The figure shows three views and two pictorial views of one solid part (mm, origin at its lowest corner). Answer the questions. Round coordinates to 2 decimals unless told otherwise and drop trailing zeros. Order: outer loops, then holes, each group sorted by start corner. A loop starts at its lowest first (then second) coordinate and runs counter-clockwise, first axis right, second up. Notation, with made-up numbers: (54.25, 88.25) - (81.25, 88.25) arc R22 ccw to (81.25, 96.25) - close; hole circle Ø1 at (17, 39). An arc over 180 degrees is marked (long way). Use CSV: the item, a comma, the result in double quotes. Start each with the question number.
Item 1: Find section B-B, the plane y = 44. Give the vertices of the cut face in (x, z).
Item 2: Find section A-A, the plane z = 0.65. Give the vertices of the cut face in (x, y), plus the area to 3 significant figures.
Item 3: Find section C-C, the plane x = 65. Give the vertices of the cut face in (y, z).
Item 4: Straight lines are drawn through the part: line 1 along X through (y, z) = (45, 2.55); line 2 along X through (y, z) = (63.5, 0.6); line 3 along Y through (x, z) = (15, 3.05). For each, find the intervals that lie inside material, in ascending order. Write a range as [from, to].
Item 5: Find section D-D, the plane y = 63.5. Give the vertices of the cut face in (x, z), plus the area to 3 significant figures.
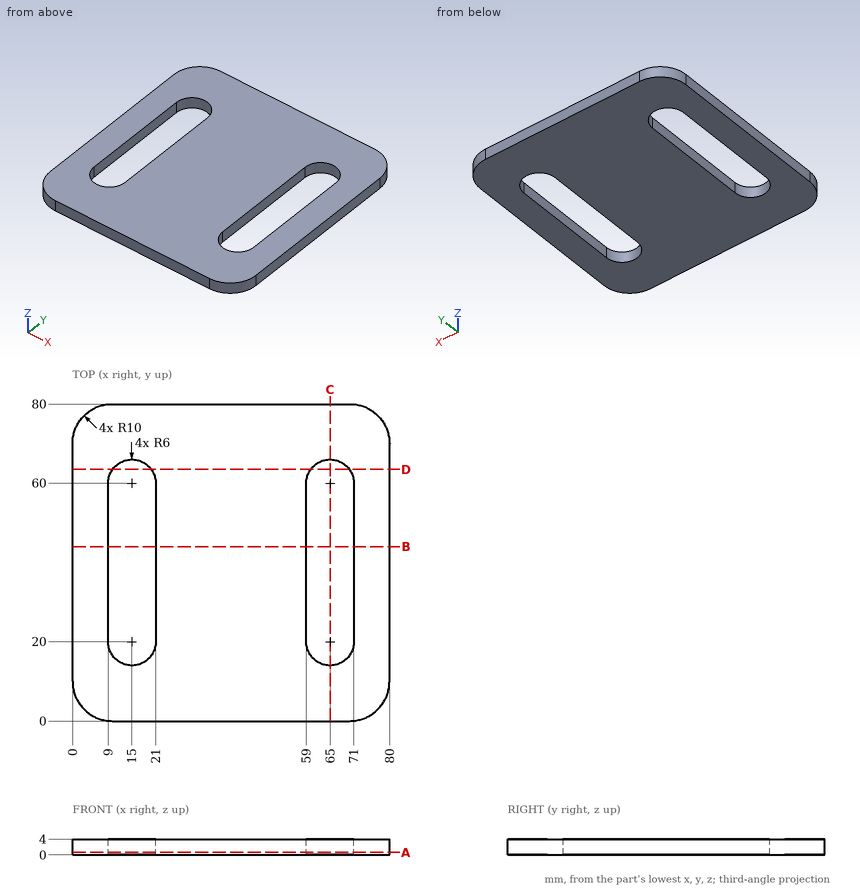
Worked out:
1,outline,"(0, 0) - (9, 0) - (9, 4) - (0, 4) - close; (21, 0) - (59, 0) - (59, 4) - (21, 4) - close; (71, 0) - (80, 0) - (80, 4) - (71, 4) - close"
2,outline,"(0, 10) arc R10 ccw to (10, 0) - (70, 0) arc R10 ccw to (80, 10) - (80, 70) arc R10 ccw to (70, 80) - (10, 80) arc R10 ccw to (0, 70) - close; hole (9, 20) arc R6 ccw to (21, 20) - (21, 60) arc R6 ccw to (9, 60) - close; hole (59, 20) arc R6 ccw to (71, 20) - (71, 60) arc R6 ccw to (59, 60) - close"
2,area,"5,130 mm²"
3,outline,"(0, 0) - (14, 0) - (14, 4) - (0, 4) - close; (66, 0) - (80, 0) - (80, 4) - (66, 4) - close"
4,line 1,"x = [0, 9], [21, 59], [71, 80]"
4,line 2,"x = [0, 10.13], [19.87, 60.13], [69.87, 80]"
4,line 3,"y = [0, 14], [66, 80]"
5,outline,"(0, 0) - (10.13, 0) - (10.13, 4) - (0, 4) - close; (19.87, 0) - (60.13, 0) - (60.13, 4) - (19.87, 4) - close; (69.87, 0) - (80, 0) - (80, 4) - (69.87, 4) - close"
5,area,"242 mm²"
